```python
from build123d import *

# Parameters (mm, degrees)
ESQUISSE1_W                     = 31.115
ESQUISSE1_H                     = 24.13
ESQUISSE1_R                     = 0.5953125
BOSS_EXTRU_1_DEPTH              = 0.5715
ESQUISSE2_W                     = 3.81
ESQUISSE2_H                     = 1.651
BOSS_EXTRU_2_DEPTH              = 2.4765
ESQUISSE3_W                     = 0.550333333
ESQUISSE3_H                     = 0.550333334
ESQUISSE3_H_2                   = 0.550333333
BOSS_EXTRU_3_DEPTH              = 0.635
ESQUISSE9_W                     = 2.54
ESQUISSE9_H                     = 10.16
BOSS_EXTRU_6_DEPTH              = 2.667
BOSS_EXTRU_7_START              = -5.08
ESQUISSE10_W                    = 0.635
ESQUISSE10_H                    = 0.635
BOSS_EXTRU_7_DEPTH              = 10.795
ESQUISSE4_R                     = 1.27
ENL_V_MAT_EXTRU_1_DEPTH         = 0.127
ESQUISSE5_W                     = 1.796051224
ESQUISSE5_H                     = 1.796051224
ENL_V_MAT_EXTRU_2_DEPTH         = 0.127
ESQUISSE7_R                     = 2.8575
BOSS_EXTRU_4_DEPTH              = 1.143
ESQUISSE8_R                     = 2.413
BOSS_EXTRU_5_DEPTH              = 7.62
CONG_1_R                        = 2.413
CONG_1_OF_R_P_T_PAR_ESQUISSE1_R = 2.413


with BuildPart() as part:
    # Esquisse1 → Boss.-Extru.1 (new, symmetric)
    with BuildSketch(Plane(origin=(0, 0, 0), x_dir=(1, 0, 0), z_dir=(0, 1, 0))):
        Rectangle(ESQUISSE1_W, ESQUISSE1_H)
        with Locations(Location((-13.6525, 10.16, 0), (0, 0, 270))):
            Circle(ESQUISSE1_R, mode=Mode.SUBTRACT)
        with Locations(Location((13.6525, 10.16, 0), (0, 0, 270))):
            Circle(ESQUISSE1_R, mode=Mode.SUBTRACT)
        with Locations(Location((-13.6525, -10.16, 0), (0, 0, 270))):
            Circle(ESQUISSE1_R, mode=Mode.SUBTRACT)
        with Locations(Location((13.6525, -10.16, 0), (0, 0, 270))):
            Circle(ESQUISSE1_R, mode=Mode.SUBTRACT)
    extrude(amount=BOSS_EXTRU_1_DEPTH, both=True)

    # Esquisse2 → Boss.-Extru.2 (add, symmetric)
    with BuildSketch(Plane.XY):
        with Locations((0, 1.397)):
            Rectangle(ESQUISSE2_W, ESQUISSE2_H)
    extrude(amount=BOSS_EXTRU_2_DEPTH, both=True)

    # Esquisse3 → Boss.-Extru.3 (add)
    with BuildSketch(Plane(origin=(0, 0.5715, 0), x_dir=(1, 0, 0), z_dir=(0, 1, 0))):
        with Locations((2.180166666, 1.651)):
            Rectangle(ESQUISSE3_W, ESQUISSE3_H)
        with Locations((2.180166666, 0.550333334)):
            Rectangle(ESQUISSE3_W, ESQUISSE3_H_2)
        with Locations((2.180166666, -0.550333334)):
            Rectangle(ESQUISSE3_W, ESQUISSE3_H_2)
        with Locations((2.180166666, -1.651)):
            Rectangle(ESQUISSE3_W, ESQUISSE3_H)
    boss_extru_3 = extrude(amount=BOSS_EXTRU_3_DEPTH)

    # Esquisse9 → Boss.-Extru.6 (add)
    with BuildSketch(Plane.XZ.offset(0.5715)):
        with Locations((13.73, 0)):
            Rectangle(ESQUISSE9_W, ESQUISSE9_H)
    boss_extru_6 = extrude(amount=BOSS_EXTRU_6_DEPTH)

    # Esquisse10 → Boss.-Extru.7 (add)
    with BuildSketch(Plane.XZ.offset(3.2385).offset(BOSS_EXTRU_7_START)):
        with Locations((13.73, 3.81)):
            Rectangle(ESQUISSE10_W, ESQUISSE10_H)
        with Locations((13.73, 1.27)):
            Rectangle(ESQUISSE10_W, ESQUISSE10_H)
        with Locations((13.73, -1.27)):
            Rectangle(ESQUISSE10_W, ESQUISSE10_H)
        with Locations((13.73, -3.81)):
            Rectangle(ESQUISSE10_W, ESQUISSE10_H)
    boss_extru_7 = extrude(amount=BOSS_EXTRU_7_DEPTH)

    # Symétrie1: Boss.-Extru.3, Boss.-Extru.7 across plane
    add(boss_extru_3.mirror(Plane(origin=(0, 0, 0), x_dir=(0, 0, 1), z_dir=(1, 0, 0))))
    add(boss_extru_7.mirror(Plane(origin=(0, 0, 0), x_dir=(0, 0, 1), z_dir=(1, 0, 0))))

    # Symétrie2: Boss.-Extru.6 across plane
    add(boss_extru_6.mirror(Plane(origin=(0, 0, 0), x_dir=(0, 0, 1), z_dir=(1, 0, 0))))

    # Esquisse4 → Enlèv. mat.-Extru.1 (cut)
    with BuildSketch(Plane(origin=(0, 2.2225, 0), x_dir=(1, 0, 0), z_dir=(0, 1, 0))):
        with Locations(Location((0, 0, 0), (0, 0, 270))):
            Circle(ESQUISSE4_R)
    extrude(amount=-ENL_V_MAT_EXTRU_1_DEPTH, mode=Mode.SUBTRACT)

    # Esquisse5 → Enlèv. mat.-Extru.2 (cut)
    with BuildSketch(Plane(origin=(0, 2.0955, 0), x_dir=(1, 0, 0), z_dir=(0, 1, 0))):
        Rectangle(ESQUISSE5_W, ESQUISSE5_H)
    extrude(amount=-ENL_V_MAT_EXTRU_2_DEPTH, mode=Mode.SUBTRACT)

    # Esquisse7 → Boss.-Extru.4 (add)
    with BuildSketch(Plane(origin=(0, 0.5715, 0), x_dir=(1, 0, 0), z_dir=(0, 1, 0))):
        with Locations(Location((-7.6835, 8.3185, 0), (0, 0, 90))):
            Circle(ESQUISSE7_R)
    boss_extru_4 = extrude(amount=BOSS_EXTRU_4_DEPTH)

    # Esquisse8 → Boss.-Extru.5 (add)
    with BuildSketch(Plane(origin=(0, 1.7145, 0), x_dir=(1, 0, 0), z_dir=(0, 1, 0))):
        with Locations(Location((-7.6835, 8.3185, 0), (0, 0, 90))):
            Circle(ESQUISSE8_R)
    boss_extru_5 = extrude(amount=BOSS_EXTRU_5_DEPTH)

    # Congé1
    cong_1_edges = [part.edges().sort_by_distance(p)[0] for p in [
        (-7.6835, 9.3345, -5.9055),
    ]]
    fillet(cong_1_edges, radius=CONG_1_R)

    # Répét. par esquisse1: Boss.-Extru.4, Boss.-Extru.5 at 3 more places
    with Locations((15.367, 0, 0), (15.367, 0, 16.637), (0, 0, 16.637)):
        add(boss_extru_4)
        add(boss_extru_5)

    # Congé1 of Répét. par esquisse1
    cong_1_of_r_p_t_par_esquisse1_edges = [part.edges().sort_by_distance(p)[0] for p in [
        (7.6835, 9.3345, -5.9055),
        (7.6835, 9.3345, 10.7315),
        (-7.6835, 9.3345, 10.7315),
    ]]
    fillet(cong_1_of_r_p_t_par_esquisse1_edges, radius=CONG_1_OF_R_P_T_PAR_ESQUISSE1_R)


solid = part.part
```
The model under review builds one solid part; all positions refer to its coordinate system, in mm. A direction names the side the tool comes from. Give positions to 0.01 mm unless a question says otherwise; leave off trailing zeros. Write each loop counter-clockwise with the first axis right and the second up, starting at its lowest first coordinate (ties: lowest second). Pieces come first, ordered by that corner, then holes. Notation, with made-up numbers: (-31, -34.5) -> (23, -34.5) arc R17 cw to (23, -15.5) -> close; hole circle Ø7 at (56, 48). An arc over 180 degrees is marked (long way). Answer in a Markdown table with one row per item.
1) Mouldability with a two-part tool opening along Z and no side actions: class faces 4 (the flat face through (-12.46, -2, 0)), 5 (the flat face through (0, 1, -2.476)), 6 (the flat face through (-1.905, 2, 0)) as +Z half, -Z half, draft (parallel to the pull), parting line (faces both ways), or undercut.
Worked answers:
| item | result |
|---|---|
| face 4 | draft |
| face 5 | -Z half |
| face 6 | undercut |
2) Add section A-A on z = 10.16. State the section outline as (x, y) points, plus the area to 3 significant figures.
Worked answers:
| item | result |
|---|---|
| outline | (-15.56, -0.57) -> (-14.25, -0.57) -> (-14.25, 0.57) -> (-15.56, 0.57) -> close; (-13.06, -0.57) -> (13.06, -0.57) -> (13.06, 0.57) -> (9.87, 0.57) -> (9.87, 1.71) -> (9.24, 1.71) -> (9.24, 6.92) arc R1.56 ccw to (6.12, 6.92) -> (6.12, 1.71) -> (5.5, 1.71) -> (5.5, 0.57) -> (-5.5, 0.57) -> (-5.5, 1.71) -> (-6.12, 1.71) -> (-6.12, 6.92) arc R1.56 ccw to (-9.24, 6.92) -> (-9.24, 1.71) -> (-9.87, 1.71) -> (-9.87, 0.57) -> (-13.06, 0.57) -> close; (14.25, -0.57) -> (15.56, -0.57) -> (15.56, 0.57) -> (14.25, 0.57) -> close |
| area | 82.9 mm² |
3) For L1, parallel to X at y = 0.2, z = -10.16; L2, parallel to Y at x = 12.5, z = 1.75; L3, parallel to X at y = -7.5, z = -4, list the stretches that pass through material, from the lowest coordinate up. Write a range as [from, to].
Worked answers:
| item | result |
|---|---|
| L1 | [-15.56, -14.25], [-13.06, 13.06], [14.25, 15.56] |
| L2 | [-3.24, 0.57] |
| L3 | [-14.05, -13.41], [13.41, 14.05] |
4) Add section D-D on y = 3. State the section outline as (x, z) points.
Worked answers:
| item | result |
|---|---|
| outline | circle Ø4.83 at (-7.68, -8.32); circle Ø4.83 at (-7.68, 8.32); circle Ø4.83 at (7.68, -8.32); circle Ø4.83 at (7.68, 8.32) |
5) Clearance check with flat-ended pins moving along their axes: P1, Ø1, axis at y = -2, z = -1.5, coming from the +X side; P2, Ø4, axis at y = 6, z = -5.5, coming from the +X side; P3, Ø0.6, axis at x = 2, y = 1, coming from the +Z side; P4, Ø8, axis at x = 4, y = -6.5, coming from the -Z side. State where each tip first meets the part, or that it passes through.
Worked answers:
| item | result |
|---|---|
| P1 | x = 15 |
| P2 | x = 9.95 |
| P3 | z = 2.48 |
| P4 | through |
6) Add section C-C on y = 8. State the section outline as (x, z) points.
Worked answers:
| item | result |
|---|---|
| outline | circle Ø4.32 at (-7.68, -8.32); circle Ø4.32 at (-7.68, 8.32); circle Ø4.32 at (7.68, -8.32); circle Ø4.32 at (7.68, 8.32) |
7) Tool access review of faces 1 (the cylindrical face through (10.473, 1.135, 8.938)), 2 (the flat face through (0, 1, 2.476)), 3 (the flat face through (14, -2, -5.08)): name each direction out of +Z, -Z, +X, -X, +Y, -Y from which nothing blocks a thin tool from reaching the whole face with its end or side.
Worked answers:
| item | result |
|---|---|
| face 1 | +Y |
| face 2 | +Z, +X, -X, +Y |
| face 3 | -Z, +X, -X, -Y |
